from build123d import *

# Parameters (mm, degrees)
SZKIC1_R                    = 120
SZKIC1_R_2                  = 90
DODANIE_WYCI_GNI_CIE1_DEPTH = 4
DODANIE_WYCI_GNI_CIE2_START = -4
DODANIE_WYCI_GNI_CIE2_DEPTH = 8
SZYK_KO_OWY1_COUNT          = 8


with BuildPart() as part:
    # Szkic1 → Dodanie-wyciągnięcie1 (new, symmetric)
    with BuildSketch(Plane.XY):
        Circle(SZKIC1_R)
        Circle(SZKIC1_R_2, mode=Mode.SUBTRACT)
    extrude(amount=DODANIE_WYCI_GNI_CIE1_DEPTH, both=True)

    # Szkic2 → Dodanie-wyciągnięcie2 (add)
    with BuildSketch(Plane.XY.offset(DODANIE_WYCI_GNI_CIE2_START)):
        with BuildLine():
            Line((5, 75), (-5, 75))
            Line((-5, 75), (-5, 81))
            ThreePointArc((-5, 81), (-7.798428028, 87.063572066), (-14.228153471, 88.868215065))
            ThreePointArc((-14.228153471, 88.868215065), (0, 90), (14.228153471, 88.868215065))
            ThreePointArc((14.228153471, 88.868215065), (7.798428028, 87.063572066), (5, 81))
            Line((5, 81), (5, 75))
        make_face()
    dodanie_wyci_gni_cie2 = extrude(amount=DODANIE_WYCI_GNI_CIE2_DEPTH)

    # Szyk kołowy1: Dodanie-wyciągnięcie2 ×8 about axis
    szyk_ko_owy1_axis = Axis((0, 0, 0), (0, 0, 1))
    for i in range(1, SZYK_KO_OWY1_COUNT):
        add(dodanie_wyci_gni_cie2.rotate(szyk_ko_owy1_axis, i * 360 / SZYK_KO_OWY1_COUNT))


solid = part.part
Verification items for the finished model (mm, model axes). A direction names the side the tool comes from. Round coordinates to 2 decimals unless told otherwise and drop trailing zeros. Loops run counter-clockwise (first coordinate to the right, second up) from the corner with the lowest first, then second, coordinate; pieces in that order, holes last. Notation, with made-up numbers: M -8.75,27.25 L 26.25,27.25 A19 cw 26.25,53.25 Z; hole C -25,30 d8. An arc over 180 degrees is marked long. Write each question's results on one line, items separated by ' | '.
1) Section check B-B on y = 33.5. Record the boundary of the cut face in (x, z), then the cut area to 3 significant figures.
Checks:
outline: M -115.23,-4 L -83.53,-4 L -83.53,4 L -115.23,4 Z; M 83.53,-4 L 115.23,-4 L 115.23,4 L 83.53,4 Z | area: 507 mm2
2) Access from +Z, -Z, +X, -X, +Y, -Y to the whole of each face (thin tool, end or side, straight path). Record for faces 4 (the flat face through (-2, -78, -4)), 5 (the flat face through (78, -5, 0)).
Checks:
face 4: -Z, +X, -X, +Y, -Y | face 5: +Z, -Z
3) Mould release check, pull along X, two halves, no side actions. Record for faces 1 (the cylindrical face through (-87.001, -7.725, -0.056)), 2 (the cylindrical face through (-119.884, 5.276, 0.056)), 3 (the flat face through (-2, -78, 4)): released by +X, released by -X, zero draft, split by the parting line, or undercut.
Checks:
face 1: undercut | face 2: split by the parting line | face 3: zero draft
4) Section check A-A on x = 0. Record the boundary of the cut face in (y, z), then the cut area to 3 significant figures.
Checks:
outline: M -120,-4 L -75,-4 L -75,4 L -120,4 Z; M 75,-4 L 120,-4 L 120,4 L 75,4 Z | area: 720 mm2
5) Scan lines: L1, parallel to Y at x = 3, z = -1.5; L2, parallel to X at y = -53.5, z = -3.25; L3, parallel to Y at x = -80.5, z = 0.25. Record each from-to range of solid material in increasing order. Write a range as from..to.
Checks:
L1: y = -119.96..-75, 75..119.96 | L2: x = -107.41..-72.31, -60.57..-52.57, 52.57..60.57, 72.31..107.41 | L3: y = -88.99..-40.25, -5..5, 40.25..88.99
6) Gauge pin test, flat ends, axial feed: P1, Ø3, axis at y = 78.5, z = 2, coming from the -X side; P2, Ø1, axis at y = 44, z = -0.5, coming from the +X side; P3, Ø1.8, axis at y = 78, z = 0.5, coming from the +X side; P4, Ø4, axis at y = -1.5, z = -2, coming from the +X side. Record the tip position at first contact, or that the pin passes through.
Checks:
P1: stops at x = -92.04 | P2: stops at x = 111.84 | P3: stops at x = 91.95 | P4: stops at x = 120
7) Section check C-C on y = -98. Record the boundary of the cut face in (x, z), then the cut area to 3 significant figures.
Checks:
outline: M -69.25,-4 L 69.25,-4 L 69.25,4 L -69.25,4 Z | area: 1,110 mm2
